Input: dimensioned drawing with shaded views. Units: mm. Origin: part minimum x, y, z. A direction names the side the tool comes from. Coordinates: 2 decimals unless noted, no trailing zeros. Order: outer loops, then holes, each group sorted by start corner. A loop starts at its lowest first (then second) coordinate and runs counter-clockwise, first axis right, second up.
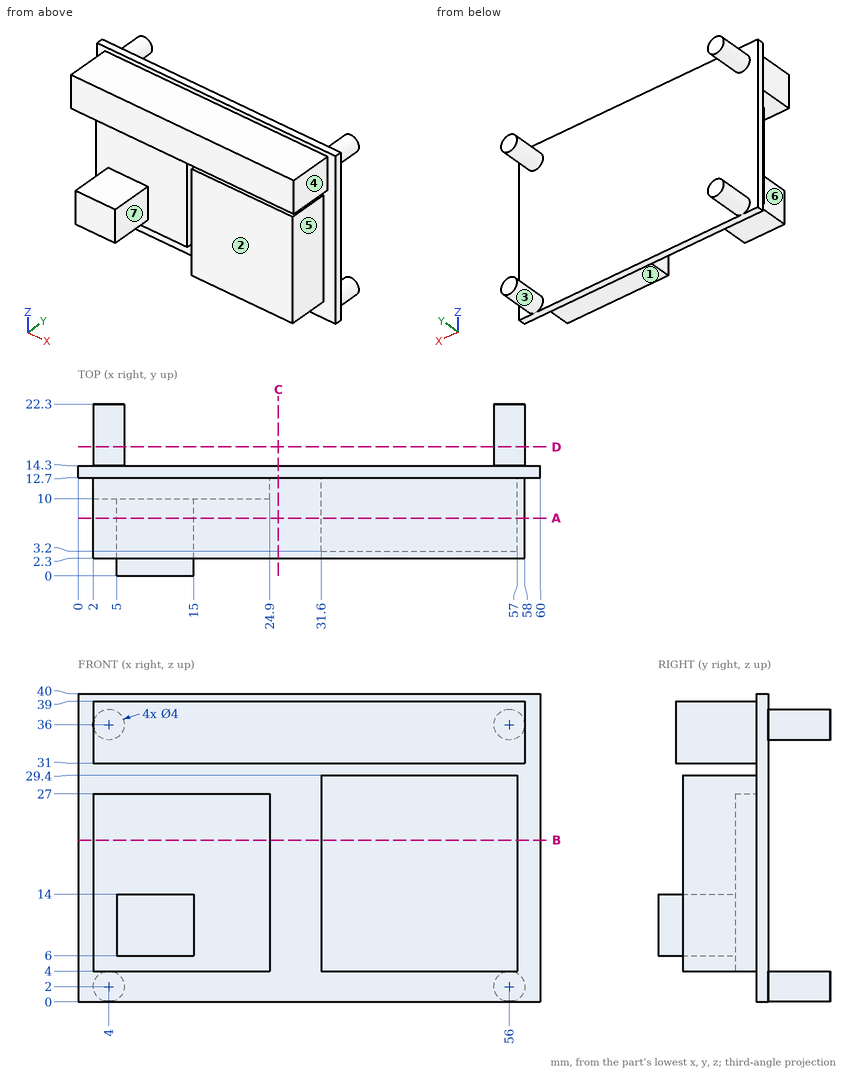
1. Section query D-D on y = 16.75. Return loops of the section in (x, z), plus the area to 3 significant figures.
Findings:
outline: circle Ø4 at (4, 2); circle Ø4 at (4, 36); circle Ø4 at (56, 2); circle Ø4 at (56, 36)
area: 50.3 mm2
2. Section query B-B on z = 21. Return loops of the section in (x, y), plus the area to 3 significant figures.
Findings:
outline: (0, 12.7) - (2, 12.7) - (2, 10) - (24.9, 10) - (24.9, 12.7) - (31.6, 12.7) - (31.6, 3.2) - (57, 3.2) - (57, 12.7) - (60, 12.7) - (60, 14.3) - (0, 14.3) - close
area: 399 mm2
3. Ray query, line 1 (Z direction, x = 4, y = 11); line 2 (Z direction, x = 11.5, y = 4.25); line 3 (Y direction, x = 56, z = 24). Return the intervals inside material, ascending.
Findings:
line 1: z = 4 to 27, 31 to 39
line 2: z = 6 to 14, 31 to 39
line 3: y = 3.2 to 14.3
4. Section query A-A on y = 7.5. Return loops of the section in (x, z), plus the area to 3 significant figures.
Findings:
outline: (2, 31) - (58, 31) - (58, 39) - (2, 39) - close; (5, 6) - (15, 6) - (15, 14) - (5, 14) - close; (31.6, 4) - (57, 4) - (57, 29.4) - (31.6, 29.4) - close
area: 1,170 mm2
5. Section query C-C on x = 26. Return loops of the section in (y, z).
Findings:
outline: (2.3, 31) - (12.7, 31) - (12.7, 0) - (14.3, 0) - (14.3, 40) - (12.7, 40) - (12.7, 39) - (2.3, 39) - close
6. Access query for the marked faces 4, 5, 6 and 7. Directions: +Z, -Z, +X, -X, +Y, -Y. A direction counts if a zero-diameter tool reaches every point of the face in a straight line with its end or side. Return the directions, or none.
Findings:
face 4: +Z, -Z, +X, -Y
face 5: -Z, +X, -Y
face 6: -Z, -X, -Y
face 7: -Z, -Y
7. Pin query (flat end, axial travel): P1, Ø3, axis at x = 35.5, y = 7, coming from the -Z side; P2, Ø6, axis at x = 27.5, z = 11.5, coming from the -Y side; P3, Ø9, axis at y = 7, z = 8, coming from the +X side; P4, Ø12, axis at x = 31, y = 7.5, coming from the -Z side. Return the tip coordinate at first contact, or that it passes through.
Findings:
P1: stops at z = 4
P2: stops at y = 10
P3: stops at x = 57
P4: stops at z = 0
8. Draft query along Z for the marked faces 1, 2 and 3. Return one class per face: released by +Z, released by -Z, zero draft, split by the parting line, or undercut.
Findings:
face 1: released by -Z
face 2: zero draft
face 3: undercut
